Design review of the part built by this model. Coordinates are the model's own, in mm. Face numbers are marked on the shaded views. A direction names the side the tool comes from. Coordinates: 2 decimals unless noted, no trailing zeros. Write each loop counter-clockwise with the first axis right and the second up, starting at its lowest first coordinate (ties: lowest second). Pieces come first, ordered by that corner, then holes.
Q1. Take a section at C-C (x = 17). Give the boundary of the cut face in (y, z).
Q2. Take a section at B-B (z = -3). Give the boundary of the cut face in (x, y), and give its area (3 significant figures).
Q3. For probe 1 along Z at (x, y) = (17, 4.4); probe 2 along X at (y, z) = (1.25, -3.25); probe 3 along Y at (x, z) = (15.75, -3.5), list the stretches that pass through material, from the lowest coordinate up.
Q4. Take a section at A-A (y = 3.75). Give the boundary of the cut face in (x, z).
Q5. Insertion check: pin 1 (3 mm diameter, centred on x = 3.5, z = -3.5, fed in from +Y); pin 2 (2.5 mm diameter, centred on x = 3, z = -3, fed in from +Y); pin 3 (2 mm diameter, centred on x = 4.5, z = -1.5, fed in from +Y). Each pin has a flat end and moves straight along its axis. Give the tip position at first contact, or say it passes through.
Q6. Machinability: for the marked faces 4 and 5, which of the approach directions +Z, -Z, +X, -X, +Y, -Y give a long, thin tool a straight path to every point of the face, cutting with its end or side? Answer none if there is none.
Q7. Take a section at D-D (y = 1). Give the boundary of the cut face in (x, z).
Q8. Mouldability with a two-part tool opening along Z and no side actions: class the marked faces 1, 2 and 3 as pulls with the +Z half, pulls with the -Z half, needs draft (parallel to the pull), parting line crosses it, or undercut.
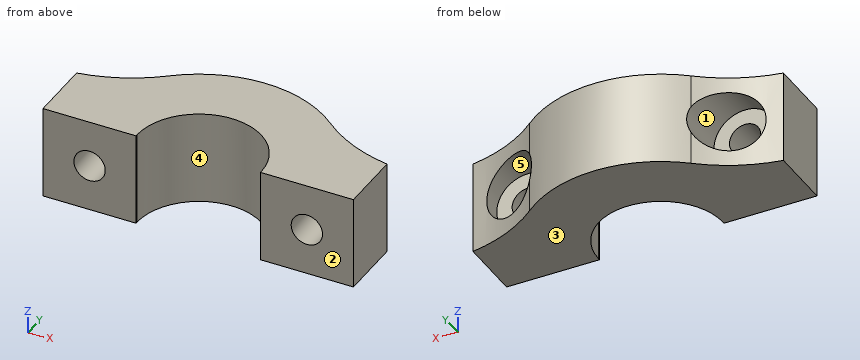
```python
from build123d import *

# Parameters (mm, degrees)
SKETCH1_W           = 20
SKETCH1_H           = 6
BOSS_EXTRUDE1_DEPTH = 4.01
BOSS_EXTRUDE2_DEPTH = 6
SKETCH5_W           = 20
SKETCH5_H           = 6
BOSS_EXTRUDE3_DEPTH = 3
SKETCH6_R           = 4.01
CUT_EXTRUDE2_DEPTH  = 8
SKETCH7_W           = 20
SKETCH7_H           = 6
CUT_EXTRUDE3_DEPTH  = 3
FILLET1_R           = 10
SKETCH8_R           = 1.01
CUT_EXTRUDE4_DEPTH  = 23.393010339
CUT_EXTRUDE5_START  = -3
SKETCH9_R           = 2
CUT_EXTRUDE5_DEPTH  = 10
BOSS_EXTRUDE4_START = 0.1
SKETCH10_W          = 5.99
SKETCH10_H          = 6
SKETCH10_R          = 1.01
BOSS_EXTRUDE4_DEPTH = 0.1


with BuildPart() as part:
    # Sketch1 → Boss-Extrude1 (new body)
    with BuildSketch(Plane(origin=(0, 0, 0), x_dir=(1, 0, 0), z_dir=(0, 1, 0))):
        with Locations((10, 3)):
            Rectangle(SKETCH1_W, SKETCH1_H)
    extrude(amount=BOSS_EXTRUDE1_DEPTH)

    # Sketch2 → Boss-Extrude2 (add)
    with BuildSketch(Plane.XY):
        with BuildLine():
            Line((2.973847991, 4.01), (17.026152009, 4.01))
            ThreePointArc((17.026152009, 4.01), (10, 8.089926579), (2.973847991, 4.01))
        make_face()
    extrude(amount=-BOSS_EXTRUDE2_DEPTH)

    # Sketch5 → Boss-Extrude3 (add)
    with BuildSketch(Plane.XZ):
        with Locations((10, -3)):
            Rectangle(SKETCH5_W, SKETCH5_H)
    extrude(amount=BOSS_EXTRUDE3_DEPTH)

    # Sketch6 → Cut-Extrude2 (cut)
    with BuildSketch(Plane.XY):
        with Locations((10, 0)):
            Circle(SKETCH6_R)
    extrude(amount=-CUT_EXTRUDE2_DEPTH, mode=Mode.SUBTRACT)

    # Sketch7 → Cut-Extrude3 (cut)
    with BuildSketch(Plane.XZ.offset(3)):
        with Locations((10, -3)):
            Rectangle(SKETCH7_W, SKETCH7_H)
    extrude(amount=-CUT_EXTRUDE3_DEPTH, mode=Mode.SUBTRACT)

    # Fillet1
    # the kernel refuses this fillet: 10 mm, written as the material it adds along each edge
    with BuildSketch(Plane(origin=(17.026152009, 4.01, 0), x_dir=(1, 0, 0), z_dir=(0, 0, -1))) as fillet1_piece_1:
        with BuildLine():
            CenterArc((4.573770937, -9.871182633), FILLET1_R, 99.206448973, 30.677642317)
            Line((-1.838595026, -2.197750365), (-1.966842345, -2.04428172))
            ThreePointArc((-1.966842345, -2.04428172), (-0.974617613, -1.052595468), (-0.173701255, 0.099135634))
            Line((-0.173701255, 0.099135634), (0, 0.2))
            ThreePointArc((0, 0.2), (1.486923995, 0.2), (2.941849532, 0.197423653))
            Line((2.941849532, 0.197423653), (2.973847991, 0))
        make_face()
    extrude(amount=6)
    with BuildSketch(Plane(origin=(2.973847991, 4.01, 0), x_dir=(0.6416530517809019, 0.7669950202838707, 0), z_dir=(0, 0, -1))) as fillet1_piece_2:
        with BuildLine():
            CenterArc((4.636373844, -9.841933994), FILLET1_R, 100.200714573, 30.677642317)
            Line((-1.908178639, -2.2809266), (-2.039069689, -2.129706452))
            ThreePointArc((-2.039069689, -2.129706452), (-1.107488324, -1.01213269), (-0.153399004, 0.12833061))
            Line((-0.153399004, 0.12833061), (0.035419403, 0.19683868))
            ThreePointArc((0.035419403, 0.19683868), (1.432701848, 0.072125761), (2.829984292, 0.19683868))
            Line((2.829984292, 0.19683868), (2.865403695, 0))
        make_face()
    extrude(amount=6)

    # Sketch8 → Cut-Extrude4 (cut, through all)
    with BuildSketch(Plane.XZ):
        with Locations(Location((3, -3, 0), (0, 0, 270))):
            Circle(SKETCH8_R)
        with Locations(Location((17, -3, 0), (0, 0, 270))):
            Circle(SKETCH8_R)
    extrude(amount=-CUT_EXTRUDE4_DEPTH, mode=Mode.SUBTRACT)

    # Sketch9 → Cut-Extrude5 (cut)
    with BuildSketch(Plane.XZ.offset(CUT_EXTRUDE5_START)):
        with Locations(Location((3, -3, 0), (0, 0, 270))):
            Circle(SKETCH9_R)
        with Locations(Location((17, -3, 0), (0, 0, 270))):
            Circle(SKETCH9_R)
    extrude(amount=-CUT_EXTRUDE5_DEPTH, mode=Mode.SUBTRACT)

    # Sketch10 → Boss-Extrude4 (add)
    # profile 1 of 2: a face of its own
    with BuildSketch(Plane.XZ.offset(BOSS_EXTRUDE4_START)):
        with Locations((2.995, -3)):
            Rectangle(SKETCH10_W, SKETCH10_H)
        with Locations(Location((3, -3, 0), (0, 0, 270))):
            Circle(SKETCH10_R, mode=Mode.SUBTRACT)
    # profile 2 of 2: a face of its own
    with BuildSketch(Plane.XZ.offset(BOSS_EXTRUDE4_START)):
        with Locations((17.005, -3)):
            Rectangle(SKETCH10_W, SKETCH10_H)
        with Locations(Location((17, -3, 0), (0, 0, 270))):
            Circle(SKETCH10_R, mode=Mode.SUBTRACT)
    extrude(amount=-BOSS_EXTRUDE4_DEPTH)


solid = part.part
```
Response:
1. outline: (-0.1, -6) - (5, -6) - (5, -5) - (3, -5) - (3, -4.01) - (-0.1, -4.01) - close; (-0.1, -1.99) - (3, -1.99) - (3, -1) - (5, -1) - (5, 0) - (-0.1, 0) - close
2. outline: (0, -0.1) - (1.99, -0.1) - (1.99, 3) - (1, 3) - (1, 4.23) arc R10 cw to (0, 4.01) - close; (4.01, -0.1) - (5.99, -0.1) - (5.99, 0) arc R4.01 cw to (14.01, 0) - (14.01, -0.1) - (15.99, -0.1) - (15.99, 3) - (15, 3) - (15, 6.36) arc R8.09 ccw to (5, 6.36) - (5, 3) - (4.01, 3) - close; (18.01, -0.1) - (20, -0.1) - (20, 4.01) arc R10 cw to (19, 4.23) - (19, 3) - (18.01, 3) - close
2. area: 71.0 mm2
3. probe 1: z = -6 to -5, -1 to 0
3. probe 2: x = 0 to 2.02, 3.98 to 6.19, 13.81 to 16.02, 17.98 to 20
3. probe 3: y = -0.1 to 3
4. outline: (0, -6) - (8.58, -6) - (8.58, 0) - (0, 0) - close; (11.42, -6) - (20, -6) - (20, 0) - (11.42, 0) - close; hole circle Ø4 at (3, -3); hole circle Ø4 at (17, -3)
5. pin 1: stops at y = 6.36
5. pin 2: stops at y = 3
5. pin 3: stops at y = 6.72
6. face 4: +Z, -Z, -Y
6. face 5: +Y
7. outline: (0, -6) - (6.12, -6) - (6.12, 0) - (0, 0) - close; (13.88, -6) - (20, -6) - (20, 0) - (13.88, 0) - close; hole circle Ø2.02 at (3, -3); hole circle Ø2.02 at (17, -3)
8. face 1: undercut
8. face 2: needs draft
8. face 3: pulls with the -Z half
